from build123d import *

# Parameters (mm, degrees)
SKETCH1_R           = 8.25
BOSS_EXTRUDE1_DEPTH = 36
BOSS_EXTRUDE1_DRAFT = -3
CUT_EXTRUDE1_DEPTH  = 3
CUT_EXTRUDE2_DEPTH  = 23
FILLET1_R           = 1


with BuildPart() as part:
    # Sketch1 → Boss-Extrude1 (with draft: the straight prism first)
    with BuildSketch(Plane(origin=(0, 0, 0), x_dir=(1, 0, 0), z_dir=(0, 1, 0))):
        Circle(SKETCH1_R)
    extrude(amount=BOSS_EXTRUDE1_DEPTH)
    # Boss-Extrude1: the draft: its side faces are tilted about the plane it starts from
    boss_extrude1_sides = [part.faces().sort_by_distance(p)[0] for p in [
        (-8.25, 18, 0),
    ]]
    draft(boss_extrude1_sides, Plane(origin=(0, 0, 0), x_dir=(1, 0, 0), z_dir=(0, 1, 0)), BOSS_EXTRUDE1_DRAFT)

    # Sketch2 → Cut-Extrude1 (cut, symmetric)
    with BuildSketch(Plane(origin=(0, 0, 0), x_dir=(0, 0, -1), z_dir=(1, 0, 0))):
        with BuildLine():
            Line((-5, 0), (5, 0))
            Line((5, 0), (5, 25))
            ThreePointArc((5, 25), (0, 30), (-5, 25))
            Line((-5, 25), (-5, 0))
        make_face()
    extrude(amount=CUT_EXTRUDE1_DEPTH, both=True, mode=Mode.SUBTRACT)

    # Sketch3 → Cut-Extrude2 (cut, symmetric)
    with BuildSketch(Plane.XY):
        Polygon((-5, 0), (5, 0), (13.833076703, 8.833076703), (13.833076703, -5.869531207), (-13.833076703, -5.869531207), (-13.833076703, 8.833076703), align=None)
    extrude(amount=CUT_EXTRUDE2_DEPTH, both=True, mode=Mode.SUBTRACT)

    # Fillet1
    fillet1_edges = [part.edges().sort_by_distance(p)[0] for p in [
        (-10.136680054, 36, 0),
    ]]
    fillet(fillet1_edges, radius=FILLET1_R)


solid = part.part
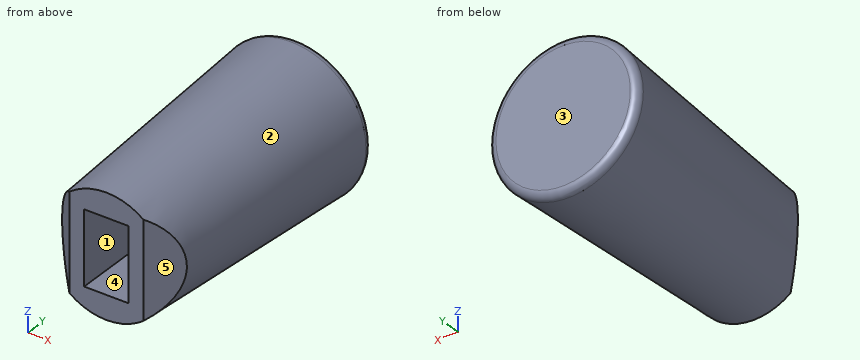
Can you work these out from the model? Positions are in its coordinate system, mm. Face numbers are marked on the shaded views. A direction names the side the tool comes from. Give positions to 0.01 mm unless a question says otherwise; leave off trailing zeros. Loops run counter-clockwise (first coordinate to the right, second up) from the corner with the lowest first, then second, coordinate; pieces in that order, holes last. Notation, with made-up numbers: (8.25, 88) - (50.25, 88) arc R16 cw to (50.25, 110) - close; hole circle Ø7 at (42.5, 4.25). An arc over 180 degrees is marked (long way). Return JSON: item names as keys, results as strings.
1. I'm going to push flat-ended pins straight in: pin 1 Ø3 at (x, y) = (1, 18) entering from -Z; pin 2 Ø3 at (y, z) = (16, -2) entering from -X; pin 3 Ø6 at (y, z) = (19.5, 8) entering from +X. Where does each tip first touch, or does it pass through?
Output values:
{"pin 1": "stops at z = -9.26", "pin 2": "stops at x = -9.1", "pin 3": "stops at x = 7.82"}
2. We'd pull the mould along X, two halves only. Please class the marked faces 1, 2 and 3: +X half, -X half, draft (parallel to the pull), parting line (faces both ways), or undercut.
Output values:
{"face 1": "undercut", "face 2": "parting line", "face 3": "draft"}
3. I want a section at A-A on y = 3. Please give me the cut outline in (x, z), and give its area (3 significant figures).
Output values:
{"outline": "(-8, -2.58) arc R8.41 ccw to (8, -2.58) - (8, 2.58) arc R8.41 ccw to (-8, 2.58) - close; hole (-3, -5) - (3, -5) - (3, 5) - (-3, 5) - close", "area": "159 mm²"}
4. I want a section at C-C on y = 16.5. Please give me the cut outline in (x, z).
Output values:
{"outline": "circle Ø18.23 at (0, 0); hole (-3, -5) - (3, -5) - (3, 5) - (-3, 5) - close"}
5. I want a section at B-B on x = 0. Please give me the cut outline in (y, z).
Output values:
{"outline": "(0, -8.25) - (34.95, -10.08) arc R1 ccw to (36, -9.08) - (36, 9.08) arc R1 ccw to (34.95, 10.08) - (0, 8.25) - (0, 5) - (25, 5) arc R5 cw to (25, -5) - (0, -5) - close"}
6. For the marked faces 4 and 5, which set-ups out of +Z, -Z, +X, -X, +Y, -Y let a thin tool reach every point of the face, with its end or its side?
Output values:
{"face 4": "-Y", "face 5": "+Z, -Z, +X, -Y"}
7. I want a section at D-D on y = 30.5. Please give me the cut outline in (x, z).
Output values:
{"outline": "circle Ø19.7 at (0, 0)"}
8. If I drill on line 1 (X direction, y = 2.5, z = 3.75); line 2 (X direction, y = 25.5, z = -4.25); line 3 (Z direction, x = 0.25, y = 25), over which ranges is the centre line in solid material (lowest first)?
Output values:
{"line 1": "x = -7.5 to -3, 3 to 7.5", "line 2": "x = -8.59 to -3, 3 to 8.59", "line 3": "z = -9.56 to -5, 5 to 9.56"}
